from build123d import *

# Parameters (mm, degrees)
F1_DEPTH = 25.4
F2_R     = 5.08


with BuildPart() as f1:
    # F0 (on Top) → F1 (new body)
    with BuildSketch(Plane.XY):
        with BuildLine():
            Line((76.2, 0), (0, 0))
            Line((0, 0), (0, 114.3))
            add(Edge.make_bspline(
                [(0, 114.3), (-197.334433, 129.25868), (-63.5, -77.519546)],
                knots=[6.229935, 6.229935, 6.229935, 8.598, 8.598, 8.598], degree=2, weights=[1, 0.377193, 1]))
            Line((-63.5, -77.519546), (-63.5, -36.650248))
            Line((-63.5, -36.650248), (63.5, -36.650248))
            Line((63.5, -36.650248), (63.5, -61.713303))
            add(Edge.make_bspline(
                [(63.5, -61.713303), (76.2, -33.499707), (76.2, 0)],
                knots=[4.142951, 4.142951, 4.142951, 4.712389, 4.712389, 4.712389], degree=2, weights=[1, 0.959741, 1]))
        make_face()
        with BuildLine():
            Line((0, 114.3), (0, 0))
            Line((0, 0), (76.2, 0))
            add(Edge.make_bspline(
                [(76.2, 0), (76.2, 108.523758), (0, 114.3)],
                knots=[4.712389, 4.712389, 4.712389, 6.229935, 6.229935, 6.229935], degree=2, weights=[1, 0.725681, 1]))
        make_face()
        with BuildLine():
            Line((63.5, -115.662508), (63.5, -61.713303))
            add(Edge.make_bspline(
                [(-63.5, -77.519546), (7.208762, -186.766711), (63.5, -61.713303)],
                knots=[2.314815, 2.314815, 2.314815, 4.142951, 4.142951, 4.142951], degree=2, weights=[1, 0.610529, 1]))
            Line((-63.5, -77.519546), (-63.5, -115.662508))
            Line((-63.5, -115.662508), (63.5, -115.662508))
        make_face()
        with BuildLine():
            add(Edge.make_bspline(
                [(-63.5, -77.519546), (7.208762, -186.766711), (63.5, -61.713303)],
                knots=[2.314815, 2.314815, 2.314815, 4.142951, 4.142951, 4.142951], degree=2, weights=[1, 0.610529, 1]))
            Line((63.5, -61.713303), (63.5, -36.650248))
            Line((63.5, -36.650248), (-63.5, -36.650248))
            Line((-63.5, -36.650248), (-63.5, -77.519546))
        make_face()
    extrude(amount=F1_DEPTH)

    # F2
    f2_edges = [f1.edges().sort_by_distance(p)[0] for p in [
        (63.5, -115.662508, 12.7),
        (-63.5, -115.662508, 12.7),
        (-80.161297, 38.167571, 0),
        (-80.161297, 38.167571, 25.4),
        (0, -115.662508, 25.4),
        (-63.5, -96.591027, 0),
        (-63.5, -96.591027, 25.4),
        (63.5, -61.713303, 12.7),
        (-63.5, -77.519546, 12.7),
        (63.5, -88.687906, 0),
        (63.5, -88.687906, 25.4),
    ]]
    fillet(f2_edges, radius=F2_R)


solid = f1.part
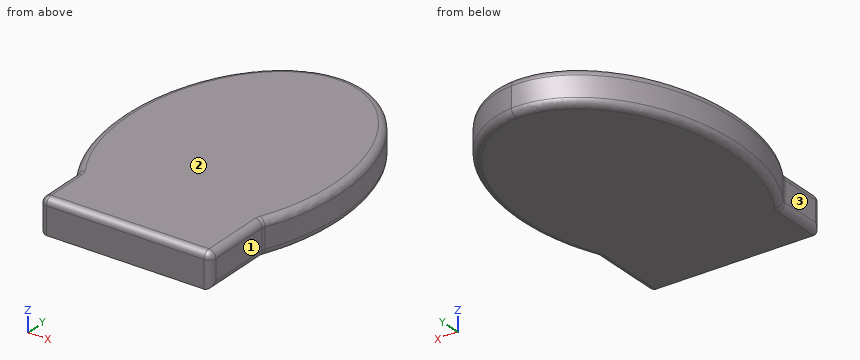
Verification items for the finished model (mm, model axes). Face numbers are marked on the shaded views. A direction names the side the tool comes from. Coordinates: 2 decimals unless noted, no trailing zeros. Loops run counter-clockwise (first coordinate to the right, second up) from the corner with the lowest first, then second, coordinate; pieces in that order, holes last. Notation, with made-up numbers: M -6.75,-28.5 L 32.25,-28.5 A21 cw 32.25,-24.5 Z; hole C -35,-0.75 d6. An arc over 180 degrees is marked long. One line per item, written item: value.
1. Section check A-A on y = -85.5. Record the cut outline in (x, z), plus the area to 3 significant figures.
Answers follow:
outline: M -63.5,5.08 A5.08 ccw -58.42,0 L 58.42,0 A5.08 ccw 63.5,5.08 L 63.5,20.32 A5.08 ccw 58.42,25.4 L -58.42,25.4 A5.08 ccw -63.5,20.32 Z
area: 3,200 mm^2
2. Gauge pin test, flat ends, axial feed: P1, Ø4, axis at y = -80.5, z = 7.5, coming from the +X side; P2, Ø10, axis at x = 49, y = 88.5, coming from the -Z side; P3, Ø8, axis at x = -15, z = 8.5, coming from the +Y side. Record the tip position at first contact, or that the pin passes through.
Answers follow:
P1: x = 63.5
P2: z = 0.33
P3: y = 114.06
3. Set-up check for the marked faces 1, 2 and 3: record each of +Z, -Z, +X, -X, +Y, -Y from which the full face is reachable in a straight line by a thin tool's end or side.
Answers follow:
face 1: +Z, -Z, +X, -Y
face 2: +Z, +X, -X, +Y, -Y
face 3: +Z, -Z, -X, -Y
4. Material ranges on line 1 along Y through (x, z) = (19.5, 11.25); line 2 along Y through (x, z) = (-16, 14.5); line 3 along X through (y, z) = (-77, 10), recorded low to high. Write a range as from..to.
Answers follow:
line 1: -115.66..109.35
line 2: -115.66..113.24
line 3: -63.91..63.5
